Part model, mm, in its own coordinate system. Round coordinates to 2 decimals unless told otherwise and drop trailing zeros. Loops run counter-clockwise (first coordinate to the right, second up) from the corner with the lowest first, then second, coordinate; pieces in that order, holes last.
1) Band-saw the part on B-B, the plane y = -70. Write the cut outline in (x, z).
2) Probe line 1 (Y direction, x = 0, z = 16); line 2 (Y direction, x = 11, z = 7); line 3 (X direction, y = -75, z = 5). List the from-to ranges inside material, lowest first.
3) Band-saw the part on D-D, the plane y = 63. Write the cut outline in (x, z).
4) Band-saw the part on A-A, the plane x = 0. Write the cut outline in (y, z).
5) Mould opens along Y. For faces 1 (the cylindrical face through (-1.953, -60.134, 17.255)), 2 (the cylindrical face through (0.573, -108.562, 17.255)), 3 (the flat face through (1, 4, 35)) say: +Y half, -Y half, draft (parallel to the pull), parting line (faces both ways), or undercut.
6) Drop flat-ended pins along their axis: P1, Ø3, axis at x = -25.5, z = 8.5, coming from the -Y side; P2, Ø8, axis at x = 2, z = 14.5, coming from the -Y side; P3, Ø6, axis at x = -28.5, z = 31, coming from the +Y side. Give the stop position or say it passes through.
7) Band-saw the part on C-C, the plane z = 6. Write the cut outline in (x, y).
from build123d import *

# Parameters (mm, degrees)
BOSS_EXTRUDE1_DEPTH     = 35
CUT_EXTRUDE1_DEPTH      = 125.410698055
CUT_EXTRUDE1_DEPTH_BACK = 125.410698055
SKETCH2_R               = 15
CUT_EXTRUDE2_DEPTH      = 125.410698055
CUT_EXTRUDE2_DEPTH_BACK = 125.410698055
SKETCH3_R               = 15


with BuildPart() as part:
    # Sketch1 → Boss-Extrude1 (new body)
    with BuildSketch(Plane.XY):
        with BuildLine():
            Line((-40, -101.071410351), (-40, 104.993508703))
            ThreePointArc((-40, 104.993508703), (0, 112.485651488), (40, 104.993508703))
            Line((40, 104.993508703), (40, -101.071410351))
            ThreePointArc((40, -101.071410351), (0, -108.563553136), (-40, -101.071410351))
        make_face()
    extrude(amount=BOSS_EXTRUDE1_DEPTH)

    # Sketch2 → Cut-Extrude1 (cut, two sides: drawn at the far end of the back side and taken through both)
    with BuildSketch(Plane.XY.offset(-CUT_EXTRUDE1_DEPTH_BACK)):
        with Locations((0, 74.993508703)):
            Circle(SKETCH2_R)
    extrude(amount=CUT_EXTRUDE1_DEPTH + CUT_EXTRUDE1_DEPTH_BACK, mode=Mode.SUBTRACT)

    # Sketch3 → Cut-Extrude2 (cut, two sides: drawn at the far end of the back side and taken through both)
    with BuildSketch(Plane.XY.offset(-CUT_EXTRUDE2_DEPTH_BACK)):
        with Locations((0, -75.006491297)):
            Circle(SKETCH3_R)
    extrude(amount=CUT_EXTRUDE2_DEPTH + CUT_EXTRUDE2_DEPTH_BACK, mode=Mode.SUBTRACT)


solid = part.part
Reported:
1. outline: (-40, 0) - (-14.14, 0) - (-14.14, 35) - (-40, 35) - close; (14.14, 0) - (40, 0) - (40, 35) - (14.14, 35) - close
2. line 1: y = -108.56 to -90.01, -60.01 to 59.99, 89.99 to 112.49
2. line 2: y = -108.01 to -85.2, -64.81 to 64.8, 85.19 to 111.94
2. line 3: x = -40 to -15, 15 to 40
3. outline: (-40, 0) - (-9.01, 0) - (-9.01, 35) - (-40, 35) - close; (9.01, 0) - (40, 0) - (40, 35) - (9.01, 35) - close
4. outline: (-108.56, 0) - (-90.01, 0) - (-90.01, 35) - (-108.56, 35) - close; (-60.01, 0) - (59.99, 0) - (59.99, 35) - (-60.01, 35) - close; (89.99, 0) - (112.49, 0) - (112.49, 35) - (89.99, 35) - close
5. face 1: undercut
5. face 2: -Y half
5. face 3: draft
6. P1: stops at y = -105.93
6. P2: stops at y = -108.56
6. P3: stops at y = 109.5
7. outline: (-40, -101.07) arc R110.52 ccw to (40, -101.07) - (40, 104.99) arc R110.52 ccw to (-40, 104.99) - close; hole circle Ø30 at (0, -75.01); hole circle Ø30 at (0, 74.99)
